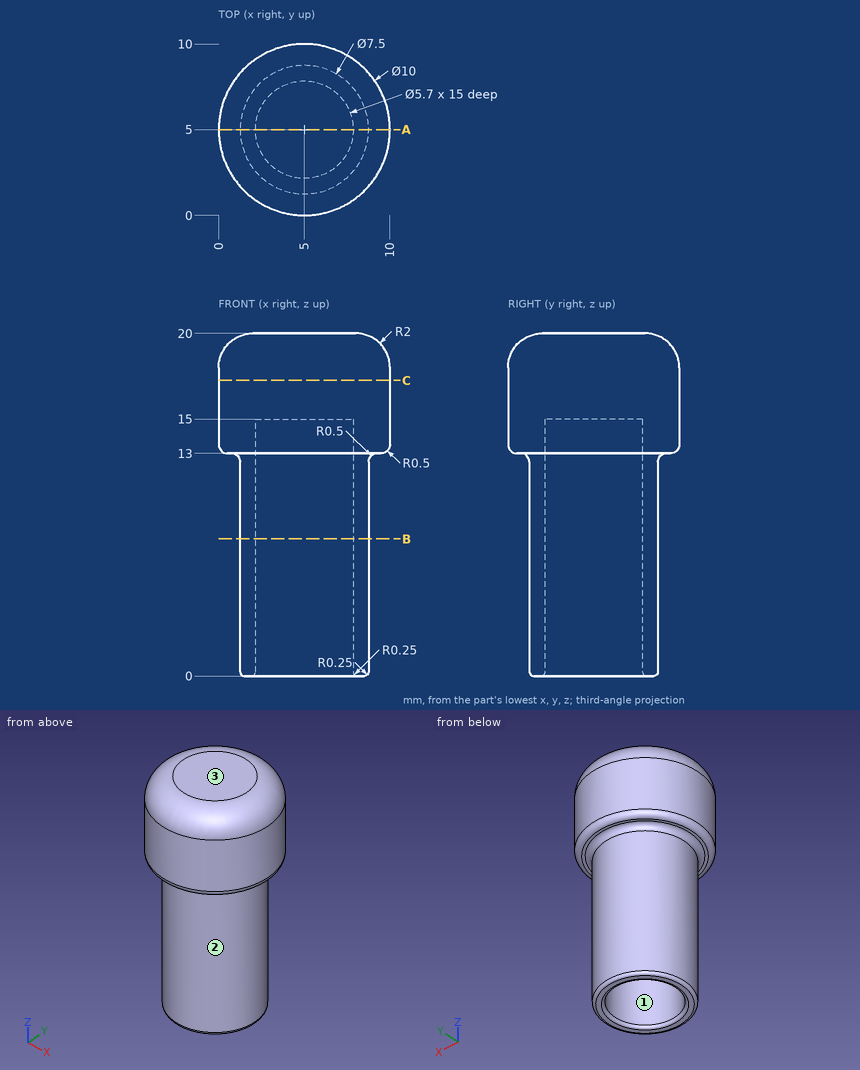
Design review of the part shown in the three views and the two pictorial views. Dimensions are in mm from the part's minimum x, y and z. Give positions to 0.01 mm unless a question says otherwise; leave off trailing zeros. Write each loop counter-clockwise with the first axis right and the second up, starting at its lowest first coordinate (ties: lowest second). Pieces come first, ordered by that corner, then holes. Notation, with made-up numbers: M 7,17.5 L 60,17.5 A10 ccw 60,35.5 Z; hole C 25.5,81 d11. An arc over 180 degrees is marked long. Answer as CSV lines item,"result".
1. Consider section C-C, the plane z = 17.25. Write out the cut boundary in (x, y), then the cut area to 3 significant figures.
Findings:
outline,"C 5,5 d10"
area,"78.5 mm2"
2. Consider section B-B, the plane z = 8. Write out the cut boundary in (x, y), then the cut area to 3 significant figures.
Findings:
outline,"C 5,5 d7.5; hole C 5,5 d5.7"
area,"18.7 mm2"
3. Draft analysis for pull direction X (two halves, no side actions). For the marked faces 1, 2 and 3, state which applies: +X half, -X half, draft (parallel to the pull), parting line (faces both ways), or undercut.
Findings:
face 1,"undercut"
face 2,"parting line"
face 3,"draft"
4. Wall thickness on line 1 (Y direction, x = 5, z = 4); line 2 (X direction, y = 1, z = 17.75); line 3 (Z direction, x = 3.25, y = 7): over which ranges is each line inside the solid? List them lowest first.
Findings:
line 1,"y = 1.25 to 2.15, 7.85 to 8.75"
line 2,"x = 2 to 8"
line 3,"z = 15 to 20"
5. For pin 1 (5 mm diameter, centred on y = 2.5, z = 5.5, fed in from -X); pin 2 (4 mm diameter, centred on x = 6, z = 6, fed in from -Y); pin 3 (1.7 mm diameter, centred on x = 5, y = 5, fed in from -Z), all flat-tipped, find the tip position at first contact; note any pin that passes through.
Findings:
pin 1,"stops at x = 1.25"
pin 2,"stops at y = 1.25"
pin 3,"stops at z = 15"
6. Consider section A-A, the plane y = 5. Write out the cut boundary in (x, z), then the cut area to 3 significant figures.
Findings:
outline,"M 0,13.5 A0.5 ccw 0.5,13 L 0.75,13 A0.5 cw 1.25,12.5 L 1.25,0.25 A0.25 ccw 1.5,0 L 1.9,0 A0.25 ccw 2.15,0.25 L 2.15,15 L 7.85,15 L 7.85,0.25 A0.25 ccw 8.1,0 L 8.5,0 A0.25 ccw 8.75,0.25 L 8.75,12.5 A0.5 cw 9.25,13 L 9.5,13 A0.5 ccw 10,13.5 L 10,18 A2 ccw 8,20 L 2,20 A2 ccw 0,18 Z"
area,"80.2 mm2"
